Check sheet for the modelled part. Datum: model origin and axes. Units: mm. Round coordinates to 2 decimals unless told otherwise and drop trailing zeros. Order: outer loops, then holes, each group sorted by start corner. A loop starts at its lowest first (then second) coordinate and runs counter-clockwise, first axis right, second up. Notation, with made-up numbers: (-14.5, 44) -> (10.5, 44) arc R9 ccw to (10.5, 58) -> close; hole circle Ø5 at (20, -33.75). An arc over 180 degrees is marked (long way). Answer as CSV lines item,"result". Start each with the question number.
from build123d import *

# Parameters (mm, degrees)
SKETCH5_R           = 15
SKETCH5_R_2         = 10
SKETCH5_R_3         = 1.5
BOSS_EXTRUDE1_DEPTH = 10


with BuildPart() as part:
    # Sketch5 → Boss-Extrude1 (new body)
    # profile 1 of 2: a face of its own
    with BuildSketch(Plane.XY):
        Polygon((-349.776309557, -150.606198532), (-449.776309557, -323.811279288), (-469.776309557, -323.811279288), (-569.776309557, -150.606198532), (-569.776309557, -20.606198532), (-349.776309557, -20.606198532), align=None)
        with Locations((-459.807870528, -262.585944494)):
            Circle(SKETCH5_R, mode=Mode.SUBTRACT)
        with Locations((-511.769394755, -172.585944494)):
            Circle(SKETCH5_R, mode=Mode.SUBTRACT)
        with Locations((-459.807870528, -202.585944494)):
            Circle(SKETCH5_R_2, mode=Mode.SUBTRACT)
        with Locations((-407.846346301, -172.585944494)):
            Circle(SKETCH5_R, mode=Mode.SUBTRACT)
    # profile 2 of 2: a face of its own
    with BuildSketch(Plane.XY):
        with Locations((-459.807870528, -202.585944494)):
            Circle(SKETCH5_R_2)
        with Locations((-464.790983154, -205.927888323)):
            Circle(SKETCH5_R_3, mode=Mode.SUBTRACT)
        with Locations((-456.465926699, -207.56905712)):
            Circle(SKETCH5_R_3, mode=Mode.SUBTRACT)
        with Locations((-454.824757902, -199.244000664)):
            Circle(SKETCH5_R_3, mode=Mode.SUBTRACT)
        with Locations((-463.149814357, -197.602831868)):
            Circle(SKETCH5_R_3, mode=Mode.SUBTRACT)
    extrude(amount=BOSS_EXTRUDE1_DEPTH)


solid = part.part
1) Depth check by flat-ended pin: pin 1 Ø1.5 at (y, z) = (-192.5, 3) entering from -X; pin 2 Ø4 at (y, z) = (-177.5, 4) entering from +X; pin 3 Ø2 at (y, z) = (-168, 3) entering from -X. Enter the tip coordinate at first touch or a pass-through.
2) Section check C-C on z = 2. Record the cut outline in (x, y).
3) Mould release check, pull along X, two halves, no side actions. Record for faces 1 (the face through (-461, -20.606, 5)), 2 (the face through (-452.9, -275.9, 4.9)), 3 (the face through (-519.076, -238.421, 4.93)): released by +X, released by -X, zero draft, split by the parting line, or undercut.
4) Section check D-D on y = -254.5. Record the cut outline in (x, z).
5) Material ranges on line 1 along X through (y, z) = (-172, 4.25); line 2 along Y through (x, z) = (-498, 4.25); line 3 along X through (y, z) = (-267, 2.5), recorded low to high.
6) Section check B-B on x = -510.5. Record the cut outline in (y, z).
7) Section check A-A on y = -176.5. Record the cut outline in (x, z), then the cut area to 3 significant figures.
Solutions:
1,pin 1,"stops at x = -546.02"
1,pin 2,"stops at x = -364.15"
1,pin 3,"stops at x = -560.31"
2,outline,"(-569.78, -150.61) -> (-469.78, -323.81) -> (-449.78, -323.81) -> (-349.78, -150.61) -> (-349.78, -20.61) -> (-569.78, -20.61) -> close; hole circle Ø30 at (-511.77, -172.59); hole circle Ø30 at (-459.81, -262.59); hole circle Ø3 at (-464.79, -205.93); hole circle Ø3 at (-463.15, -197.6); hole circle Ø3 at (-456.47, -207.57); hole circle Ø3 at (-454.82, -199.24); hole circle Ø30 at (-407.85, -172.59)"
3,face 1,"zero draft"
3,face 2,"undercut"
3,face 3,"released by -X"
4,outline,"(-509.79, 0) -> (-472.44, 0) -> (-472.44, 10) -> (-509.79, 10) -> close; (-447.17, 0) -> (-409.76, 0) -> (-409.76, 10) -> (-447.17, 10) -> close"
5,line 1,"x = -557.42 to -526.76, -496.78 to -422.83, -392.86 to -362.13"
5,line 2,"y = -274.93 to -178.54, -166.64 to -20.61"
5,line 3,"x = -502.58 to -474.14, -445.47 to -416.98"
6,outline,"(-253.28, 0) -> (-187.53, 0) -> (-187.53, 10) -> (-253.28, 10) -> close; (-157.64, 0) -> (-20.61, 0) -> (-20.61, 10) -> (-157.64, 10) -> close"
7,outline,"(-554.83, 0) -> (-526.25, 0) -> (-526.25, 10) -> (-554.83, 10) -> close; (-497.29, 0) -> (-422.33, 0) -> (-422.33, 10) -> (-497.29, 10) -> close; (-393.37, 0) -> (-364.73, 0) -> (-364.73, 10) -> (-393.37, 10) -> close"
7,area,"1,320 mm^2"
